Check sheet for the modelled part. Datum: model origin and axes. Units: mm. Face numbers are marked on the shaded views. A direction names the side the tool comes from. Round coordinates to 2 decimals unless told otherwise and drop trailing zeros. Write each loop counter-clockwise with the first axis right and the second up, starting at its lowest first coordinate (ties: lowest second). Pieces come first, ordered by that corner, then holes. Notation, with made-up numbers: M -3.5,41.25 L 38.5,41.25 A26 cw 38.5,62.25 Z; hole C 8,81.5 d3. An arc over 180 degrees is marked long. Answer in a Markdown table with one row per item.
Autodesk Inventor part; units mm, degrees
ref_plane "YZ Plane" through (0, 0, 0) normal (1, 0, 0) x (0, 1, 0)
ref_plane "XZ Plane" through (0, 0, 0) normal (0, 1, 0) x (-1, 0, 0)
ref_plane "XY Plane" through (0, 0, 0) normal (0, 0, 1) x (1, 0, 0)
sketch "Sketch1" plane through (0, 0, 0) normal (0, 0, 1) x (1, 0, 0)
  line L0 (-40.485, -25.075) -> (40.485, -25.075)
  line L1 (40.485, -25.075) -> (40.485, 25.075)
  line L2 (40.485, 25.075) -> (-40.485, 25.075)
  line L3 (-40.485, 25.075) -> (-40.485, -25.075)
  line L4 (-40.485, -25.075) -> (40.485, 25.075) construction
  line L5 (40.485, -25.075) -> (-40.485, 25.075) construction
  circle A0 centre (-37.975, 22.565) radius 1.65
  line L6 (-39.625, 24.215) -> (-36.325, 24.215) construction
  line L7 (-36.325, 24.215) -> (-36.325, 20.915) construction
  line L8 (-36.325, 20.915) -> (-39.625, 20.915) construction
  line L9 (-39.625, 20.915) -> (-39.625, 24.215) construction
  line L10 (-39.625, 24.215) -> (-36.325, 20.915) construction
  line L11 (-36.325, 24.215) -> (-39.625, 20.915) construction
  line L12 (-40.485, 0) -> (40.485, 0) construction
  line L13 (0, 25.075) -> (0, -25.075) construction
  circle A1 centre (-37.975, -22.565) radius 1.65
  line L14 (0, -25.075) -> (0, 25.075) construction
  circle A2 centre (37.975, 22.565) radius 1.65 construction
  circle A3 centre (37.975, -22.565) radius 1.65
  line L15 (37.975, 25.075) -> (37.975, 13.575) construction
  circle A4 centre (37.975, 13.575) radius 1.65
  point P0 (0, 0)
  dimension "d0" = 80.97
  dimension "d1" = 50.15
  dimension "d2" = 3.3
  dimension "d3" = 0.86
  dimension "d4" = 0.86
  dimension "d10" = 11.5
extrude "Extrusion1" add sketch "Sketch1" along normal blind 1.17
sketch "Sketch2" plane through (0, 0, 1.17) normal (0, 0, 1) x (1, 0, 0)
  line L0 (40.485, -25.075) -> (40.485, 25.075)
  line L1 (40.485, -20.075) -> (30.485, -20.075)
  line L2 (30.485, -20.075) -> (30.485, 10.275)
  line L3 (30.485, 10.275) -> (40.485, 10.275)
  line L4 (40.485, 10.275) -> (40.485, -20.075)
  line L5 (-40.485, -25.075) -> (40.485, -25.075)
  point P0 (0, 0)
  dimension "d7" = 5
  dimension "d8" = 30.35
  dimension "d9" = 10
extrude "Extrusion2" add sketch "Sketch2" along normal blind 14
sketch "Sketch3" plane through (0, 0, 1.17) normal (0, 0, 1) x (1, 0, 0)
  line L0 (40.485, 10.275) -> (40.485, 25.075) construction
  line L1 (40.485, 25.075) -> (-40.485, 25.075) construction
  circle A0 centre (35.485, 20.075) radius 5
  point P0 (0, 0)
  dimension "d13" = 10
extrude "Extrusion3" add sketch "Sketch3" along normal blind 21
fillet "Fillet1" radius 1 1 edges at (30.485, 20.075, 22.17)
sketch "Sketch4" plane through (30.485, -20.075, 1.17) normal (0, -1, 0) x (1, 0, 0)
  line L0 (0, 14) -> (10, 14) construction
  line L1 (0, 0) -> (0, 14)
  line L2 (10, 0) -> (10, 14)
  line L3 (10, 14) -> (0, 14)
  line L4 (2.5, 14) -> (8.5, 14)
  line L5 (10, 8) -> (8.5, 14)
  line L6 (2.5, 14) -> (0, 8)
  line L7 (10, 8) -> (0, 8) construction
  point P0 (-30.485, -1.17)
  dimension "d17" = 6
  dimension "d18" = 6
  dimension "d19" = 1.5
extrude "Extrusion4" cut sketch "Sketch4" against normal up to surface (30.35 mm away)
sketch "Sketch5" plane through (0, 0, 15.17) normal (0, 0, 1) x (1, 0, 0)
  line L0 (38.985, 10.275) -> (32.985, 10.275) construction
  line L1 (35.985, 10.275) -> (35.985, -20.075) construction
  line L2 (32.985, -20.075) -> (38.985, -20.075) construction
  line L3 (35.985, -20.075) -> (35.985, 10.275) construction
  circle A0 centre (35.985, 6.6536) radius 1.925
  circle A1 centre (35.985, 2.0321) radius 1.925
  circle A2 centre (35.985, -2.5893) radius 1.925
  circle A3 centre (35.985, -7.2107) radius 1.925
  circle A4 centre (35.985, -11.8321) radius 1.925
  circle A5 centre (35.985, -16.4536) radius 1.925
  point P0 (0, 0)
  dimension "d22" = 3.85
  dimension "d23" = 4.6214
  dimension "d24" = 4.6214
  dimension "d25" = 4.6214
  dimension "d26" = 4.6214
  dimension "d27" = 4.6214
  dimension "d28" = 3.6214
  dimension "d29" = 3.6214
extrude "Extrusion5" cut sketch "Sketch5" against normal blind 3.85
sketch "Sketch6" plane through (0, 0, 1.17) normal (0, 0, 1) x (1, 0, 0)
  line L0 (-25.015, 25.075) -> (25.985, 25.075)
  line L1 (25.985, 25.075) -> (25.985, -25.075)
  line L2 (25.985, -25.075) -> (-25.015, -25.075)
  line L3 (-25.015, -25.075) -> (-25.015, 25.075)
  line L4 (40.485, -25.075) -> (40.485, -20.075)
  line L5 (35.485, 25.075) -> (-40.485, 25.075)
  line L6 (-40.485, -25.075) -> (40.485, -25.075)
  point P0 (0, 0)
  dimension "d32" = 14.5
  dimension "d33" = 51
extrude "Extrusion6" add sketch "Sketch6" along normal blind 29
sketch "Sketch7" plane through (0, 0, 30.17) normal (0, 0, 1) x (1, 0, 0)
  line L0 (25.985, 25.075) -> (-25.015, 25.075)
  line L1 (-25.015, -25.075) -> (25.985, -25.075)
  line L2 (22.985, 25.075) -> (18.985, 25.075)
  line L3 (18.985, 25.075) -> (18.985, -25.075)
  line L4 (18.985, -25.075) -> (22.985, -25.075)
  line L5 (22.985, -25.075) -> (22.985, 25.075)
  line L6 (25.985, -25.075) -> (25.985, 25.075)
  line L7 (16.985, 25.075) -> (16.985, -25.075)
  line L8 (12.985, 25.075) -> (12.985, -25.075)
  line L9 (10.985, 25.075) -> (10.985, -25.075)
  line L10 (6.985, 25.075) -> (6.985, -25.075)
  line L11 (4.985, 25.075) -> (4.985, -25.075)
  line L12 (0.985, 25.075) -> (0.985, -25.075)
  line L13 (-1.015, 25.075) -> (-1.015, -25.075)
  line L14 (-5.015, 25.075) -> (-5.015, -25.075)
  line L15 (-7.015, 25.075) -> (-7.015, -25.075)
  line L16 (-11.015, 25.075) -> (-11.015, -25.075)
  line L17 (-13.015, 25.075) -> (-13.015, -25.075)
  line L18 (-17.015, 25.075) -> (-17.015, -25.075)
  line L19 (-19.015, 25.075) -> (-19.015, -25.075)
  line L20 (-23.015, 25.075) -> (-23.015, -25.075)
  point P0 (0, 0)
  dimension "d36" = 3
  dimension "d37" = 4
  dimension "d38" = 2
  dimension "d39" = 4
  dimension "d40" = 2
  dimension "d41" = 4
  dimension "d42" = 2
  dimension "d43" = 4
  dimension "d44" = 2
  dimension "d45" = 4
  dimension "d46" = 2
  dimension "d47" = 4
  dimension "d48" = 2
  dimension "d49" = 4
  dimension "d50" = 2
  dimension "d51" = 4
extrude "Extrusion7" cut sketch "Sketch7" against normal blind 25 contours L5 L1 L3 L0 | L7 L1 L8 L0 | L9 L1 L10 L0 | L11 L1 L12 L0 | L13 L1 L14 L0 | L15 L1 L16 L0 | L17 L1 L18 L0 | L19 L1 L20 L0
sketch "Sketch8" plane through (0, 0, 1.17) normal (0, 0, 1) x (1, 0, 0)
  line L0 (32.985, -20.075) -> (38.985, -20.075)
  line L1 (30.485, -20.075) -> (-40.485, -20.075) construction
  line L2 (-40.485, 25.075) -> (-40.485, -25.075)
  line L3 (-40.485, -20.075) -> (-30.485, -20.075)
  line L4 (-30.485, -20.075) -> (-30.485, -0.075)
  line L5 (-30.485, -0.075) -> (-40.485, -0.075)
  line L6 (-40.485, -0.075) -> (-40.485, -20.075)
  line L7 (40.485, 10.275) -> (40.485, -20.075)
  line L8 (30.485, -20.075) -> (30.485, 10.275)
  point P0 (0, 0)
  point P1 (-30.485, -10.075)
  dimension "d54" = 20
  dimension "d55" = 10
  dimension "d56" = 10
extrude "Extrusion8" add sketch "Sketch8" along normal up to surface (14 mm away)
sketch "Sketch10" plane through (-40.485, -20.075, 1.17) normal (0, -1, 0) x (1, 0, 0)
  line L0 (10, 14) -> (0, 14)
  line L1 (2.6888, 14) -> (7.5, 14)
  line L2 (10, 0) -> (10, 14)
  line L3 (10, 8) -> (7.5, 14)
  line L4 (0, 0) -> (0, 14)
  line L5 (1.5, 14) -> (0, 8)
  line L6 (73.47, 14) -> (79.47, 14)
  line L7 (80.97, 8) -> (79.47, 14)
  line L8 (73.47, 14) -> (70.97, 8)
  point P0 (40.485, -1.17)
  point P1 (76.47, 14)
  dimension "d59" = 1.5
  dimension "d60" = 1.5
  dimension "d61" = 2.5
  dimension "d62" = 2.5
  dimension "d63" = 6
  dimension "d64" = 6
  dimension "d65" = 6
extrude "Extrusion9" cut sketch "Sketch10" against normal up to surface (20 mm away)
sketch "Sketch11" plane through (-38.985, -0.075, 15.17) normal (0, 0, 1) x (1, 0, 0)
  line L0 (0, 0) -> (6, 0) construction
  line L1 (6, -20) -> (0, -20) construction
  line L2 (3, 0) -> (3, -20) construction
  circle A0 centre (3, -3) radius 1.925
  circle A1 centre (3, -7.6667) radius 1.925
  circle A2 centre (3, -12.3333) radius 1.925
  circle A3 centre (3, -17) radius 1.925
  circle A4 centre (74.97, 6.7286) radius 1.925
  point P0 (38.985, 0.075)
  dimension "d68" = 3
  dimension "d69" = 3
  dimension "d70" = 4.6667
  dimension "d71" = 4.6667
  dimension "d73" = 4.6667
extrude "Extrusion10" cut sketch "Sketch11" against normal blind 10 contours A0 | A1 | A2 | A3
equation "\"d24\" = d23"
equation "\"d25\" = d23"
equation "\"d26\" = d23"
equation "\"d27\" = d23"
equation "\"d30\" = d22"
equation "\"d39\" = d37"
equation "\"d40\" = d38"
equation "\"d41\" = d37"
equation "\"d42\" = d38"
equation "\"d43\" = d37"
equation "\"d44\" = d38"
equation "\"d45\" = d37"
equation "\"d46\" = d38"
equation "\"d47\" = d37"
equation "\"d48\" = d38"
equation "\"d49\" = d37"
equation "\"d50\" = d38"
equation "\"d51\" = d37"
equation "\"d60\" = d59"
equation "\"d62\" = d61"
equation "\"d64\" = d63"
equation "\"d65\" = d63"
equation "\"d71\" = d70"
equation "\"d73\" = d70"
properties part number "HiLetgoTB6600HG"
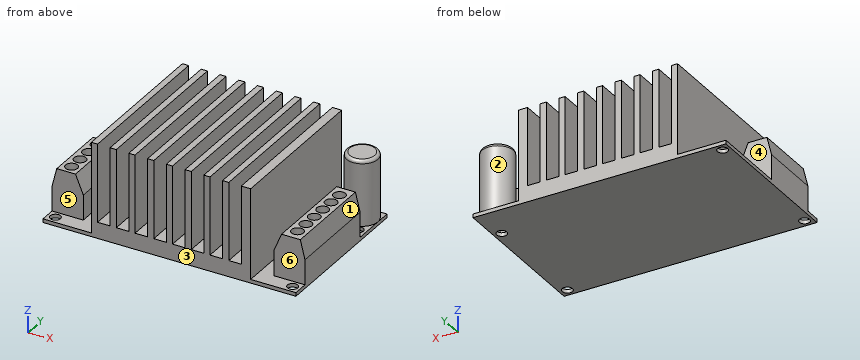
1. Go/stop test with flat-tipped pins: pin 1 (12 mm diameter, centred on x = 16.5, z = 17.5, fed in from -Y) (3 decimals); pin 2 (1.2 mm diameter, centred on x = -36.5, y = -16.5, fed in from +Z); pin 3 (3 mm diameter, centred on x = 36.5, y = -6.5, fed in from +Z); pin 4 (10 mm diameter, centred on y = -12.5, z = 19.5, fed in from -X). Record where each tip stops, or that it passes through.
Found:
| item | result |
|---|---|
| pin 1 | stops at y = -25.075 |
| pin 2 | stops at z = 5.17 |
| pin 3 | stops at z = 15.17 |
| pin 4 | stops at x = -39.15 |
2. Scan lines: L1, parallel to Y at x = -36, z = 12 (3 decimals); L2, parallel to X at y = -15, z = 2 (3 decimals); L3, parallel to X at y = 7.5, z = 3 (3 decimals). Record each from-to range of solid material in increasing order.
Found:
| item | result |
|---|---|
| L1 | y = -20.075 to -19, -15.15 to -14.333, -10.483 to -9.667, -5.817 to -5, -1.15 to -0.075 |
| L2 | x = -40.485 to -30.485, -25.015 to 25.985, 30.485 to 40.485 |
| L3 | x = -25.015 to 25.985, 30.485 to 40.485 |
3. Section check A-A, the plane z = 4. Record the cut outline in (x, y) (3 decimals), and give its area (3 significant figures).
Found:
| item | result |
|---|---|
| outline | M -40.485,-20.075 L -30.485,-20.075 L -30.485,-0.075 L -40.485,-0.075 Z; M -25.015,-25.075 L 25.985,-25.075 L 25.985,25.075 L -25.015,25.075 Z; M 30.485,-20.075 L 40.485,-20.075 L 40.485,10.275 L 30.485,10.275 Z; C 35.485,20.075 d10 |
| area | 3,140 mm2 |
4. Draft check along X on the marked faces 1, 2 and 3. Enter one of: +X half, -X half, draft (parallel to the pull), parting line (faces both ways), or undercut.
Found:
| item | result |
|---|---|
| face 1 | +X half |
| face 2 | undercut |
| face 3 | draft |
5. Section check B-B, the plane x = 28. Record the cut outline in (y, z) (3 decimals).
Found:
| item | result |
|---|---|
| outline | M -25.075,0 L 25.075,0 L 25.075,1.17 L -25.075,1.17 Z |
6. Access from +Z, -Z, +X, -X, +Y, -Y to the whole of each face (thin tool, end or side, straight path). Record for the marked faces 4, 5 and 6.
Found:
| item | result |
|---|---|
| face 4 | +Z, -X, +Y |
| face 5 | +Z, -X, -Y |
| face 6 | +Z, +X, -Y |
7. Section check C-C, the plane z = 26. Count the separate pieces of the cut face and the enclosed holes in it, and give its area (3 significant figures).
Found:
| item | result |
|---|---|
| separate pieces | 9 |
| enclosed holes | 0 |
| area | 953 mm2 |
